from build123d import *
from build123d.topology import SkipClean

# Parameters (mm, degrees)
SALIENTE_EXTRUIR1_DEPTH = 10
CROQUIS2_R              = 5
SALIENTE_EXTRUIR2_DEPTH = 20


with BuildPart() as part:
    # Croquis1 → Saliente-Extruir1 (new body)
    with BuildSketch(Plane(origin=(0, 0, 0), x_dir=(1, 0, 0), z_dir=(0, 1, 0))):
        with BuildLine():
            Line((-60, -34.207532581), (60, -34.207532581))
            ThreePointArc((60, -34.207532581), (65, -39.207532581), (60, -44.207532581))
            Line((60, -44.207532581), (-60, -44.207532581))
            ThreePointArc((-60, -44.207532581), (-65, -39.207532581), (-60, -34.207532581))
        make_face()
    extrude(amount=SALIENTE_EXTRUIR1_DEPTH)

    # Croquis2 → Saliente-Extruir2 (add)
    with SkipClean():  # the faces are left unmerged after this step: merging them gives an invalid solid
        with BuildSketch(Plane(origin=(0, 10, 0), x_dir=(1, 0, 0), z_dir=(0, 1, 0))):
            with Locations(Location((60, -39.207532581, 0), (0, 0, 270))):
                Circle(CROQUIS2_R)
            with Locations(Location((-60, -39.207532581, 0), (0, 0, 270))):
                Circle(CROQUIS2_R)
        extrude(amount=SALIENTE_EXTRUIR2_DEPTH)
    add(part.part.scale(1), mode=Mode.REPLACE)  # the faces are merged on a copy


solid = part.part
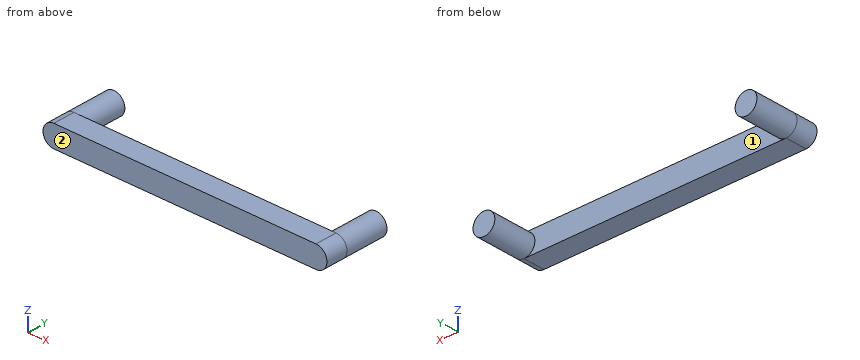
Input: part model. Units: mm. Frame: model coordinates. Face numbers are marked on the shaded views. Give positions to 0.01 mm unless a question says otherwise; leave off trailing zeros. Order: outer loops, then holes, each group sorted by start corner. A loop starts at its lowest first (then second) coordinate and runs counter-clockwise, first axis right, second up. Notation, with made-up numbers: M 79.5,9 L 120.5,9 A26 cw 120.5,46 Z; hole C 81.25,75.5 d5. An arc over 180 degrees is marked long. Answer as a JSON object with one key per item and string values.
1. First-contact query: P1, Ø4, axis at y = 26, z = 35.5, coming from the +X side; P2, Ø1.5, axis at y = 14, z = 43, coming from the +X side. Flat tips, straight axial feed; report the tip coordinate or a pass-through.
Result sheet:
{"P1": "x = 64.7", "P2": "x = 63.97"}
2. Cut plane C-C, the plane x = 37. Output: boundary loops of the cut face in (y, z).
Result sheet:
{"outline": "M 0,34.21 L 10,34.21 L 10,44.21 L 0,44.21 Z"}
3. Cut plane D-D, the plane y = 2.5. Output: boundary loops of the cut face in (x, z), and give its area (3 significant figures).
Result sheet:
{"outline": "M -60,34.21 L 60,34.21 A5 ccw 60,44.21 L -60,44.21 A5 ccw Z", "area": "1,280 mm²"}
4. Cut plane A-A, the plane y = 17. Output: boundary loops of the cut face in (x, z).
Result sheet:
{"outline": "C -60,39.21 d10; C 60,39.21 d10"}
5. Pull-direction query (X, two-part tool) for the marked faces 1 and 2; classes: +X half, -X half, draft (parallel to the pull), parting line (faces both ways), or undercut.
Result sheet:
{"face 1": "undercut", "face 2": "draft"}
6. Ray query, line 1 (Y direction, x = 35.5, z = 35.75); line 2 (X direction, y = 13.5, z = 36.5); line 3 (X direction, y = 16, z = 39.5). Return the intervals inside material, ascending. Write a range as [from, to].
Result sheet:
{"line 1": "[0, 10]", "line 2": "[-64.2, -55.8], [55.8, 64.2]", "line 3": "[-64.99, -55.01], [55.01, 64.99]"}
7. Cut plane B-B, the plane z = 41.5. Output: boundary loops of the cut face in (x, y), and give its area (3 significant figures).
Result sheet:
{"outline": "M -64.44,0 L 64.44,0 L 64.44,30 L 55.56,30 L 55.56,10 L -55.56,10 L -55.56,30 L -64.44,30 Z", "area": "1,640 mm²"}
